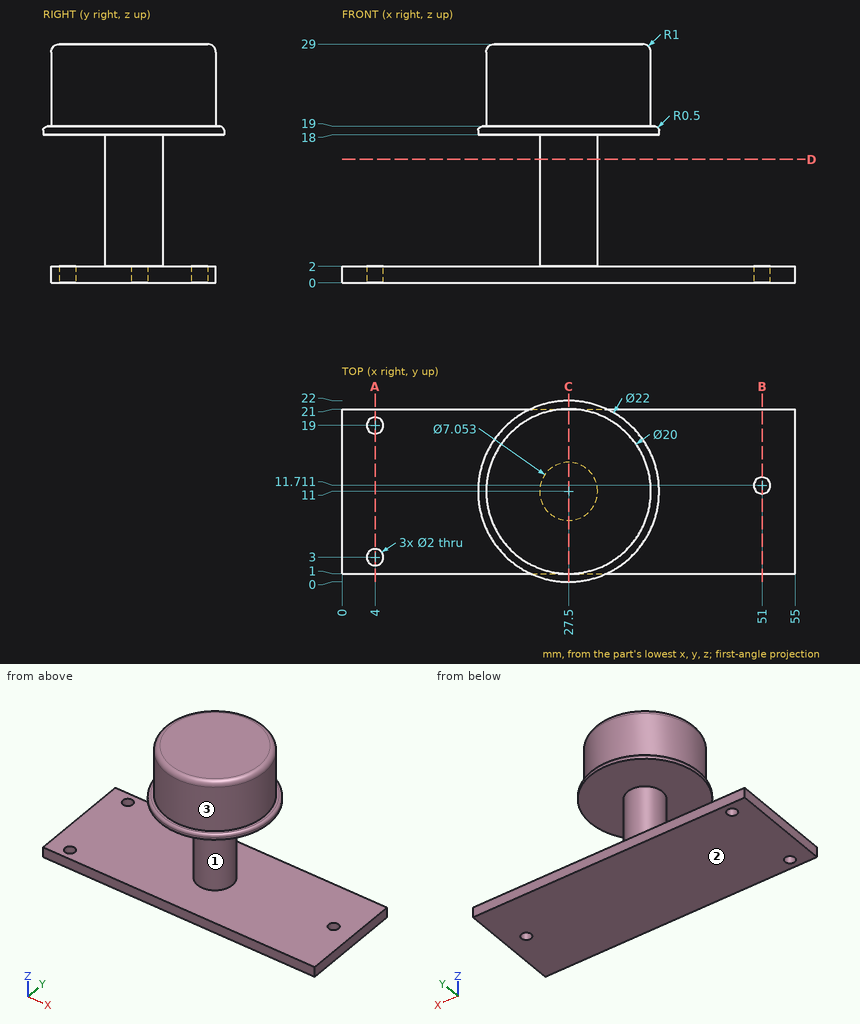
Could you check a few things on this drawing? It's one solid part, dimensions in mm from its lowest x, y, z. A direction names the side the tool comes from. Coordinates: 2 decimals unless noted, no trailing zeros. Write each loop counter-clockwise with the first axis right and the second up, starting at its lowest first coordinate (ties: lowest second). Pieces come first, ordered by that corner, then holes. Notation, with made-up numbers: (9.25, -13) - (51.25, -13) arc R31 ccw to (51.25, 21) - close; hole circle Ø4 at (16.5, 27). An arc over 180 degrees is marked (long way). Put each result on its own line as item: value. Start each with the question number.
Q1. I want a section at C-C on x = 27.5. Write out the boundary of the cut face in (y, z).
Q2. I'm going to push flat-ended pins straight in: P1, Ø3, axis at x = 4, y = 19, coming from the +Z side; P2, Ø5, axis at x = 8, y = 11, coming from the -Z side; P3, Ø12, axis at x = 28.5, z = 24.5, coming from the +Y side (1 decimal); P4, Ø2, axis at x = 27.5, z = 1, coming from the -Y side. Where does each tip first touch, or does it pass through?
Q3. I want a section at A-A on x = 4. Write out the boundary of the cut face in (y, z).
Q4. Please list where these lines run through material, in increasing order: L1, parallel to Y at x = 4, z = 1.15; L2, parallel to Y at x = 51, z = 1.3; L3, parallel to Z at x = 24, y = 5.5.
Q5. Which directions (+Z, -Z, +X, -X, +Y, -Y) give clear straight access to the entire face, cutting with the end or side of a thin tool? Please do the marked faces 1, 2 and 3.
Q6. I want a section at B-B on x = 51. Write out the boundary of the cut face in (y, z).
Q7. I want a section at D-D on z = 15. Write out the boundary of the cut face in (x, y), plus the area to 3 significant figures.
Checks:
1. outline: (0, 18) - (7.47, 18) - (7.47, 2) - (1, 2) - (1, 0) - (21, 0) - (21, 2) - (14.53, 2) - (14.53, 18) - (22, 18) - (22, 18.5) arc R0.5 ccw to (21.5, 19) - (21, 19) - (21, 28) arc R1 ccw to (20, 29) - (2, 29) arc R1 ccw to (1, 28) - (1, 19) - (0.5, 19) arc R0.5 ccw to (0, 18.5) - close
2. P1: z = 2
2. P2: z = 0
2. P3: y = 22
2. P4: y = 1
3. outline: (1, 0) - (2, 0) - (2, 2) - (1, 2) - close; (4, 0) - (18, 0) - (18, 2) - (4, 2) - close; (20, 0) - (21, 0) - (21, 2) - (20, 2) - close
4. L1: 1 to 2, 4 to 18, 20 to 21
4. L2: 1 to 10.71, 12.71 to 21
4. L3: 0 to 2, 18 to 29
5. face 1: none
5. face 2: -Z, +X, -X, +Y, -Y
5. face 3: +Z
6. outline: (1, 0) - (10.71, 0) - (10.71, 2) - (1, 2) - close; (12.71, 0) - (21, 0) - (21, 2) - (12.71, 2) - close
7. outline: circle Ø7.05 at (27.5, 11)
7. area: 39.1 mm²
